Source: CAD feature listing. Evaluate the final solid. Frame: model axes, mm. Face numbers are marked on the shaded views. A direction names the side the tool comes from. Coordinates: 2 decimals unless noted, no trailing zeros. Loops run counter-clockwise (first coordinate to the right, second up) from the corner with the lowest first, then second, coordinate; pieces in that order, holes last. Notation, with made-up numbers: (-20.75, 18) -> (4.25, 18) arc R26 cw to (4.25, 48) -> close; hole circle Ø3 at (85, 26.5). An arc over 180 degrees is marked (long way). Answer as CSV lines item,"result".
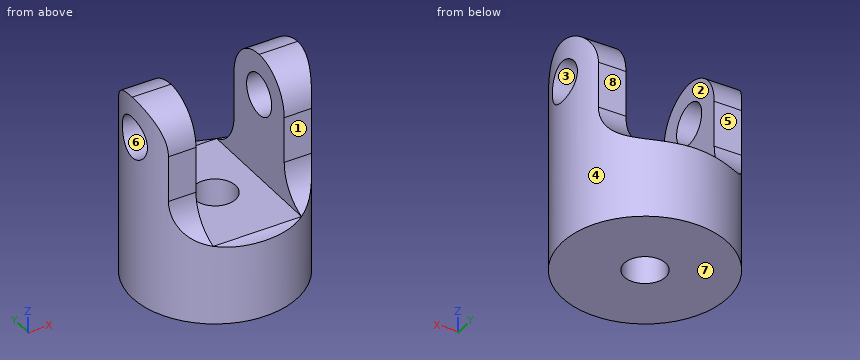
from build123d import *

# Parameters (mm, degrees)
SKETCH1_R               = 19.05
SKETCH1_R_2             = 4.765
BOSS_EXTRUDE1_DEPTH     = 47.63
CUT_EXTRUDE1_DEPTH      = 55.721311205
CUT_EXTRUDE1_DEPTH_BACK = 55.721311205
SKETCH2_W               = 20.32
SKETCH2_H               = 29.21
CUT_EXTRUDE3_DEPTH      = 55.721311205
CUT_EXTRUDE3_DEPTH_BACK = 55.721311205
CUT_EXTRUDE4_DEPTH      = 55.721311362
CUT_EXTRUDE4_DEPTH_BACK = 55.721311362


with BuildPart() as part:
    # Sketch1 → Boss-Extrude1 (new body)
    with BuildSketch(Plane.XY):
        Circle(SKETCH1_R)
        Circle(SKETCH1_R_2, mode=Mode.SUBTRACT)
    extrude(amount=BOSS_EXTRUDE1_DEPTH)

    # Sketch2 → Cut-Extrude1 (cut, two sides: drawn at the far end of the back side and taken through both)
    with BuildSketch(Plane(origin=(0, 0, 0), x_dir=(1, 0, 0), z_dir=(0, 1, 0)).offset(-CUT_EXTRUDE1_DEPTH_BACK)):
        with Locations((0, -33.025)):
            Rectangle(SKETCH2_W, SKETCH2_H)
    extrude(amount=CUT_EXTRUDE1_DEPTH + CUT_EXTRUDE1_DEPTH_BACK, mode=Mode.SUBTRACT)

    # Sketch3 → Cut-Extrude3 (cut, two sides: drawn at the far end of the back side and taken through both)
    with BuildSketch(Plane(origin=(0, 0, 0), x_dir=(0, 0, -1), z_dir=(1, 0, 0)).offset(-CUT_EXTRUDE3_DEPTH_BACK)):
        with BuildLine():
            Line((-47.63, 9.53), (-38.1, 9.53))
            Line((-38.1, 9.53), (-27.476114037, 9.53))
            ThreePointArc((-27.476114037, 9.53), (-34.545985954, 12.674475624), (-36.945471337, 20.030648934))
            Line((-36.945471337, 20.030648934), (-47.497981878, 20.575601986))
            Line((-47.497981878, 20.575601986), (-55.897546117, 9.53))
            Line((-55.897546117, 9.53), (-47.63, 9.53))
        make_face()
        with BuildLine():
            ThreePointArc((-36.945471337, 20.030648934), (-34.545985954, 12.674475624), (-27.476114037, 9.53))
            ThreePointArc((-27.476114037, 9.53), (-20.74445748, 12.318343443), (-17.956114037, 19.05))
            Line((-17.956114037, 19.05), (-36.945471337, 20.030648934))
        make_face()
        with BuildLine():
            ThreePointArc((-17.956114037, 19.05), (-26.985136182, 28.557330895), (-36.945471337, 20.030648934))
            Line((-36.945471337, 20.030648934), (-17.956114037, 19.05))
        make_face()
        with BuildLine():
            ThreePointArc((-47.63, 0), (-44.838727625, 6.738727625), (-38.1, 9.53))
            Line((-38.1, 9.53), (-47.63, 9.53))
            Line((-47.63, 9.53), (-47.63, 0))
        make_face()
        with BuildLine():
            ThreePointArc((-38.1, -9.53), (-44.838727625, -6.738727625), (-47.63, 0))
            Line((-47.63, 0), (-47.63, -9.53))
            Line((-47.63, -9.53), (-38.1, -9.53))
        make_face()
        with BuildLine():
            Line((-27.476114037, -9.53), (-38.1, -9.53))
            Line((-38.1, -9.53), (-47.63, -9.53))
            Line((-47.63, -9.53), (-55.897546117, -9.53))
            Line((-55.897546117, -9.53), (-47.497981878, -20.575601986))
            Line((-47.497981878, -20.575601986), (-36.945471337, -20.030648934))
            ThreePointArc((-36.945471337, -20.030648934), (-34.545985954, -12.674475624), (-27.476114037, -9.53))
        make_face()
        with BuildLine():
            ThreePointArc((-17.956114037, -19.05), (-20.74445748, -12.318343443), (-27.476114037, -9.53))
            ThreePointArc((-27.476114037, -9.53), (-34.545985954, -12.674475624), (-36.945471337, -20.030648934))
            Line((-36.945471337, -20.030648934), (-17.956114037, -19.05))
        make_face()
        with BuildLine():
            ThreePointArc((-36.945471337, -20.030648934), (-26.985136182, -28.557330895), (-17.956114037, -19.05))
            Line((-17.956114037, -19.05), (-36.945471337, -20.030648934))
        make_face()
    extrude(amount=CUT_EXTRUDE3_DEPTH + CUT_EXTRUDE3_DEPTH_BACK, mode=Mode.SUBTRACT)

    # Sketch3_5 → Cut-Extrude4 (cut, two sides: drawn at the far end of the back side and taken through both)
    with BuildSketch(Plane(origin=(0, 0, 0), x_dir=(0, 0, -1), z_dir=(1, 0, 0)).offset(-CUT_EXTRUDE4_DEPTH_BACK)):
        with BuildLine():
            ThreePointArc((-42.865, 0), (-38.1, -4.765), (-33.335, 0))
            Line((-33.335, 0), (-42.865, 0))
        make_face()
        with BuildLine():
            Line((-42.865, 0), (-33.335, 0))
            ThreePointArc((-33.335, 0), (-38.1, 4.765), (-42.865, 0))
        make_face()
    extrude(amount=CUT_EXTRUDE4_DEPTH + CUT_EXTRUDE4_DEPTH_BACK, mode=Mode.SUBTRACT)


solid = part.part
(1) Draft query along Y for the marked faces 6, 7 and 8. Return one class per face: released by +Y, released by -Y, zero draft, split by the parting line, or undercut.
Computed values:
face 6,"undercut"
face 7,"zero draft"
face 8,"released by +Y"
(2) Access query for the marked faces 1, 2, 3, 4 and 5. Directions: +Z, -Z, +X, -X, +Y, -Y. A direction counts if a zero-diameter tool reaches every point of the face in a straight line with its end or side. Return the directions, or none.
Computed values:
face 1,"+Z, +X, -X, -Y"
face 2,"+Z, +Y, -Y"
face 3,"+X, -X"
face 4,"+Z, -Z"
face 5,"+Z, +X, -X, +Y"
(3) Cut plane B-B (y = -1). Return the cut outline in (x, z), then the cut area to 3 significant figures.
Computed values:
outline,"(-19.02, 0) -> (-4.66, 0) -> (-4.66, 18.42) -> (-10.16, 18.42) -> (-10.16, 33.44) -> (-19.02, 33.44) -> close; (-19.02, 42.76) -> (-10.16, 42.76) -> (-10.16, 47.58) -> (-19.02, 47.58) -> close; (4.66, 0) -> (19.02, 0) -> (19.02, 33.44) -> (10.16, 33.44) -> (10.16, 18.42) -> (4.66, 18.42) -> close; (10.16, 42.76) -> (19.02, 42.76) -> (19.02, 47.58) -> (10.16, 47.58) -> close"
area,"881 mm^2"
(4) Cut plane A-A (z = 31.5). Return the cut outline in (x, y).
Computed values:
outline,"(-16.49, -9.53) -> (-10.16, -9.53) -> (-10.16, 9.53) -> (-16.49, 9.53) arc R19.05 ccw to start; (10.16, -9.53) -> (16.49, -9.53) arc R19.05 ccw to (16.49, 9.53) -> (10.16, 9.53) -> close"
(5) Material intervals for L1, parallel to Z at x = 13, y = 0 (3 decimals); L2, parallel to Y at x = 0, z = 14 (3 decimals); L3, parallel to Y at x = -16, z = 38, sorted ascending. Write a range as [from, to].
Computed values:
L1,"[0, 33.335], [42.865, 47.63]"
L2,"[-19.05, -4.765], [4.765, 19.05]"
L3,"[-9.53, -4.76], [4.76, 9.53]"
(6) Cut plane D-D (z = 11). Return the cut outline in (x, y) (3 decimals), then the cut area to 3 significant figures.
Computed values:
outline,"circle Ø38.1 at (0, 0); hole circle Ø9.53 at (0, 0)"
area,"1,070 mm^2"
(7) Cut plane C-C (x = -14). Return the cut outline in (y, z) (3 decimals), then the cut area to 3 significant figures.
Computed values:
outline,"(-12.919, 0) -> (12.919, 0) -> (12.919, 20.193) arc R9.52 cw to (9.53, 27.476) -> (9.53, 38.1) arc R9.53 ccw to (-9.53, 38.1) -> (-9.53, 27.476) arc R9.52 cw to (-12.919, 20.193) -> close; hole circle Ø9.53 at (0, 38.1)"
area,"949 mm^2"
(8) Pin query (flat end, axial travel): pin 1 Ø7 at (x, z) = (13, 34) entering from -Y; pin 2 Ø3 at (x, z) = (14.5, 30) entering from +Y; pin 3 Ø2 at (y, z) = (-8, 23.5) entering from -X. Return the tip coordinate at first contact, or that it passes through.
Computed values:
pin 1,"y = -9.53"
pin 2,"y = 9.53"
pin 3,"x = -17.72"
